```python
from build123d import *

# Parameters (mm, degrees)
ESBO_O1_R                = 1.7
RESSALTO_EXTRUS_O1_DEPTH = 6
CORTE_EXTRUS_O1_DEPTH    = 7.5


with BuildPart() as part:
    # Esboço1 → Ressalto-extrusão1 (new body)
    with BuildSketch(Plane.XY):
        with BuildLine():
            Line((10, 3.5), (-10, 3.5))
            ThreePointArc((-10, 3.5), (-13.5, 0), (-10, -3.5))
            Line((-10, -3.5), (10, -3.5))
            ThreePointArc((10, -3.5), (13.5, 0), (10, 3.5))
        make_face()
        with Locations((-10, 0)):
            Circle(ESBO_O1_R, mode=Mode.SUBTRACT)
        with Locations((10, 0)):
            Circle(ESBO_O1_R, mode=Mode.SUBTRACT)
    extrude(amount=RESSALTO_EXTRUS_O1_DEPTH)

    # Esboço2 → Corte-extrusão1 (cut, symmetric)
    with BuildSketch(Plane(origin=(0, 0, 0), x_dir=(0, 0, -1), z_dir=(1, 0, 0))):
        Polygon((0, 3.5), (-0.7, 3.1), (-0.7, 2.9), (0, 2.5), align=None)
        Polygon((0, 1.5), (-0.7, 1.1), (-0.7, 0.9), (0, 0.5), align=None)
        Polygon((0, -0.5), (-0.7, -0.9), (-0.7, -1.1), (0, -1.5), align=None)
        Polygon((0, -2.5), (-0.7, -2.9), (-0.7, -3.1), (0, -3.5), align=None)
    extrude(amount=CORTE_EXTRUS_O1_DEPTH, both=True, mode=Mode.SUBTRACT)


solid = part.part
```
Geometry check sheet. Reference: the model listing, model coordinates, mm. Round coordinates to 2 decimals unless told otherwise and drop trailing zeros. Loops run counter-clockwise (first coordinate to the right, second up) from the corner with the lowest first, then second, coordinate; pieces in that order, holes last. Notation, with made-up numbers: M -34.5,23 L 24.5,23 A22 ccw 24.5,35 Z; hole C -25,6 d8. An arc over 180 degrees is marked long. Return JSON: item names as keys, results as strings. Group by question number.
(1) Mould release check, pull along Y, two halves, no side actions. Record for faces 1 (the face through (0, 0, 0)), 2 (the face through (9.63, -1.66, 2.96)), 3 (the face through (0, -3.5, 3)): pulls with the +Y half, pulls with the -Y half, needs draft (parallel to the pull), parting line crosses it, or undercut.
(2) Scan lines: line 1 along Y through (x, z) = (10, 1.6); line 2 along X through (y, z) = (-1.5, 5.3); line 3 along X through (y, z) = (1.25, 3.6). Record each from-to range of solid material in increasing order. Write a range as [from, to].
(3) Section check A-A, the plane y = 0. Enter the section's corners in (x, z).
(4) Section check B-B, the plane x = 9. Enter the section's corners in (y, z).
(5) Go/stop test with flat-tipped pins: pin 1 (0.6 mm diameter, centred on y = -1, z = 0, fed in from -X); pin 2 (0.6 mm diameter, centred on y = 3, z = 0, fed in from +X); pin 3 (2 mm diameter, centred on y = -2.5, z = 0.5, fed in from +X); pin 4 (2 mm diameter, centred on x = -10, y = 0, fed in from +Z). Record where each tip stops, or that it passes through.
(6) Section check C-C, the plane z = 2. Enter the section's corners in (x, y), and give its area (3 significant figures).
(7) Section check D-D, the plane y = 2. Enter the section's corners in (x, z), and give its area (3 significant figures).
Data:
{
 "1": {"face 1": "needs draft", "face 2": "undercut", "face 3": "pulls with the -Y half"},
 "2": {"line 1": "[-3.5, -1.7], [1.7, 3.5]", "line 2": "[-13.16, -10.8], [-9.2, 9.2], [10.8, 13.16]", "line 3": "[-13.27, -11.15], [-8.85, 8.85], [11.15, 13.27]"},
 "3": {"outline": "M -13.5,0 L -11.7,0 L -11.7,6 L -13.5,6 Z; M -8.3,0 L 8.3,0 L 8.3,6 L -8.3,6 Z; M 11.7,0 L 13.5,0 L 13.5,6 L 11.7,6 Z"},
 "4": {"outline": "M -3.5,0 L -1.37,0 L -1.37,6 L -3.5,6 Z; M 1.37,0 L 3.5,0 L 3.5,6 L 1.37,6 Z"},
 "5": {"pin 1": "x = -13.43", "pin 2": "x = 12.23", "pin 3": "x = 13.16", "pin 4": "through"},
 "6": {"outline": "M -10,-3.5 L 10,-3.5 A3.5 ccw 10,3.5 L -10,3.5 A3.5 ccw Z; hole C -10,0 d3.4; hole C 10,0 d3.4", "area": "160 mm²"},
 "7": {"outline": "M -12.87,0 L 12.87,0 L 12.87,6 L -12.87,6 Z", "area": "154 mm²"}
}
